```python
from build123d import *

# Parameters (mm, degrees)
SKETCH1_R           = 13
SKETCH1_R_2         = 2.5
BOSS_EXTRUDE1_DEPTH = 3
SKETCH2_W           = 62
SKETCH2_H           = 45
BOSS_EXTRUDE2_DEPTH = 3
BOSS_EXTRUDE3_START = 42
BOSS_EXTRUDE3_DEPTH = 3
CUT_EXTRUDE1_REACH  = 74.732
FILLET1_R           = 5


# Read off the part's stored shape, not the designer's step: Boss-Extrude3
with BuildPart() as part:
    # Sketch1 → Boss-Extrude1 (new body)
    with BuildSketch(Plane(origin=(0, 0, 0), x_dir=(1, 0, 0), z_dir=(0, 1, 0))):
        with BuildLine():
            Line((0, 31), (45, 31))
            Line((45, 31), (45, -31))
            Line((45, -31), (0, -31))
            ThreePointArc((0, -31), (-31, 0), (0, 31))
        make_face()
        with Locations(Location((0, 0, 0), (0, 0, 270))):
            Circle(SKETCH1_R, mode=Mode.SUBTRACT)
        with Locations(Location((0, 25.5, 0), (0, 0, 270))):
            Circle(SKETCH1_R_2, mode=Mode.SUBTRACT)
        with Locations(Location((-25.5, 0, 0), (0, 0, 270))):
            Circle(SKETCH1_R_2, mode=Mode.SUBTRACT)
        with Locations(Location((0, -25.5, 0), (0, 0, 270))):
            Circle(SKETCH1_R_2, mode=Mode.SUBTRACT)
        with Locations(Location((25.5, 0, 0), (0, 0, 270))):
            Circle(SKETCH1_R_2, mode=Mode.SUBTRACT)
    extrude(amount=BOSS_EXTRUDE1_DEPTH)

    # Sketch2 → Boss-Extrude2 (add)
    with BuildSketch(Plane(origin=(45, 0, 0), x_dir=(0, 0, -1), z_dir=(1, 0, 0))):
        with Locations((0, 22.5)):
            Rectangle(SKETCH2_W, SKETCH2_H)
    extrude(amount=BOSS_EXTRUDE2_DEPTH)

    # Boss-Extrude3 outline → Boss-Extrude3 (add)
    with BuildSketch(Plane(origin=(0, 0, 0), x_dir=(1, 0, 0), z_dir=(0, 1, 0)).offset(BOSS_EXTRUDE3_START)):
        with BuildLine():
            ThreePointArc((0, 31), (-31, 0), (0, -31))
            Line((0, -31), (45, -31))
            Line((45, -31), (45, 31))
            Line((45, 31), (0, 31))
        make_face()
    extrude(amount=BOSS_EXTRUDE3_DEPTH)

    # Sketch4 → Cut-Extrude1 (cut, up to next)
    with BuildSketch(Plane(origin=(0, 45, 0), x_dir=(1, 0, 0), z_dir=(0, 1, 0)), mode=Mode.PRIVATE) as cut_extrude1_sk1:
        with BuildLine():
            Line((13, -13), (-13, -13))
            ThreePointArc((-13, -13), (-26, 0), (-13, 13))
            Line((-13, 13), (13, 13))
            ThreePointArc((13, 13), (26, 0), (13, -13))
        make_face()
    cut_extrude1_tool1 = extrude(cut_extrude1_sk1.sketch, amount=-CUT_EXTRUDE1_REACH, mode=Mode.PRIVATE) & part.part
    add(cut_extrude1_tool1.solids().sort_by_distance((0, 45, 0))[0], mode=Mode.SUBTRACT)

    # Fillet1
    fillet1_edges = [part.edges().sort_by_distance(p)[0] for p in [
        (45, 3, 0),
        (48, 0, 0),
        (48, 45, 0),
        (45, 42, 0),
    ]]
    fillet(fillet1_edges, radius=FILLET1_R)


solid = part.part
```
Verification items for the finished model (mm, model axes). A direction names the side the tool comes from. Give positions to 0.01 mm unless a question says otherwise; leave off trailing zeros. Order: outer loops, then holes, each group sorted by start corner. A loop starts at its lowest first (then second) coordinate and runs counter-clockwise, first axis right, second up. Notation, with made-up numbers: (8, 82) -> (12, 82) arc R10 cw to (12, 87) -> close; hole circle Ø5 at (2, -18). An arc over 180 degrees is marked (long way). Use a Markdown table: item, result.
1) Section check B-B, the plane z = 0. Record the boundary of the cut face in (x, y).
Results:
| item | result |
|---|---|
| outline | (-31, 0) -> (-28, 0) -> (-28, 3) -> (-31, 3) -> close; (-31, 42) -> (-26, 42) -> (-26, 45) -> (-31, 45) -> close; (-23, 0) -> (-13, 0) -> (-13, 3) -> (-23, 3) -> close; (13, 0) -> (23, 0) -> (23, 3) -> (13, 3) -> close; (26, 42) -> (40, 42) arc R5 cw to (45, 37) -> (45, 8) arc R5 cw to (40, 3) -> (28, 3) -> (28, 0) -> (43, 0) arc R5 ccw to (48, 5) -> (48, 40) arc R5 ccw to (43, 45) -> (26, 45) -> close |
2) Section check D-D, the plane z = 25.5. Record the boundary of the cut face in (x, y).
Results:
| item | result |
|---|---|
| outline | (-17.63, 0) -> (-2.5, 0) -> (-2.5, 3) -> (-17.63, 3) -> close; (-17.63, 42) -> (40, 42) arc R5 cw to (45, 37) -> (45, 8) arc R5 cw to (40, 3) -> (2.5, 3) -> (2.5, 0) -> (43, 0) arc R5 ccw to (48, 5) -> (48, 40) arc R5 ccw to (43, 45) -> (-17.63, 45) -> close |
3) Section check A-A, the plane x = 34.5. Record the boundary of the cut face in (y, z), then the cut area to 3 significant figures.
Results:
| item | result |
|---|---|
| outline | (0, -31) -> (3, -31) -> (3, 31) -> (0, 31) -> close; (42, -31) -> (45, -31) -> (45, 31) -> (42, 31) -> close |
| area | 372 mm² |
4) Depth check by flat-ended pin: pin 1 Ø18.5 at (x, z) = (5.5, -6) entering from -Y; pin 2 Ø8.5 at (y, z) = (21.5, -10) entering from -X; pin 3 Ø4 at (x, z) = (25.5, 0) entering from -Y. Enter the tip coordinate at first touch or a pass-through.
Results:
| item | result |
|---|---|
| pin 1 | y = 0 |
| pin 2 | x = 45 |
| pin 3 | y = 42 |
5) Tool access check on faces 1 (the flat face through (11.9, 42, 13.3)), 2 (the flat face through (45.4, 20.7, -31)), 3 (the cylindrical face through (-23, 1, 0)), 4 (the cylindrical face through (26, 44, 0)). Record the directions out of +Z, -Z, +X, -X, +Y, -Y that give a thin tool (end or side, any length) a straight path to the whole face; none if there is none.
Results:
| item | result |
|---|---|
| face 1 | +Z, -Z, -X |
| face 2 | -Z, +X, -X, +Y, -Y |
| face 3 | -Y |
| face 4 | +Y |
6) Mould release check, pull along Y, two halves, no side actions. Record for faces 5 (the flat face through (13, 3, -7)), 6 (the cylindrical face through (-7.91, 1.479, -10.316)), 7 (the cylindrical face through (46, 44, 0)): pulls with the +Y half, pulls with the -Y half, needs draft (parallel to the pull), parting line crosses it, or undercut.
Results:
| item | result |
|---|---|
| face 5 | undercut |
| face 6 | needs draft |
| face 7 | pulls with the +Y half |
7) Material ranges on probe 1 along Y at (x, z) = (-4.5, -25); probe 2 along X at (y, z) = (1, 0); probe 3 along Z at (x, y) = (10, 43), recorded low to high.
Results:
| item | result |
|---|---|
| probe 1 | 0 to 3, 42 to 45 |
| probe 2 | -31 to -28, -23 to -13, 13 to 23, 28 to 46 |
| probe 3 | -31 to -13, 13 to 31 |
8) Section check C-C, the plane z = -10. Record the boundary of the cut face in (x, y), then the cut area to 3 significant figures.
Results:
| item | result |
|---|---|
| outline | (-29.34, 0) -> (-8.31, 0) -> (-8.31, 3) -> (-29.34, 3) -> close; (-29.34, 42) -> (-21.31, 42) -> (-21.31, 45) -> (-29.34, 45) -> close; (8.31, 0) -> (43, 0) arc R5 ccw to (48, 5) -> (48, 40) arc R5 ccw to (43, 45) -> (21.31, 45) -> (21.31, 42) -> (40, 42) arc R5 cw to (45, 37) -> (45, 8) arc R5 cw to (40, 3) -> (8.31, 3) -> close |
| area | 403 mm² |
